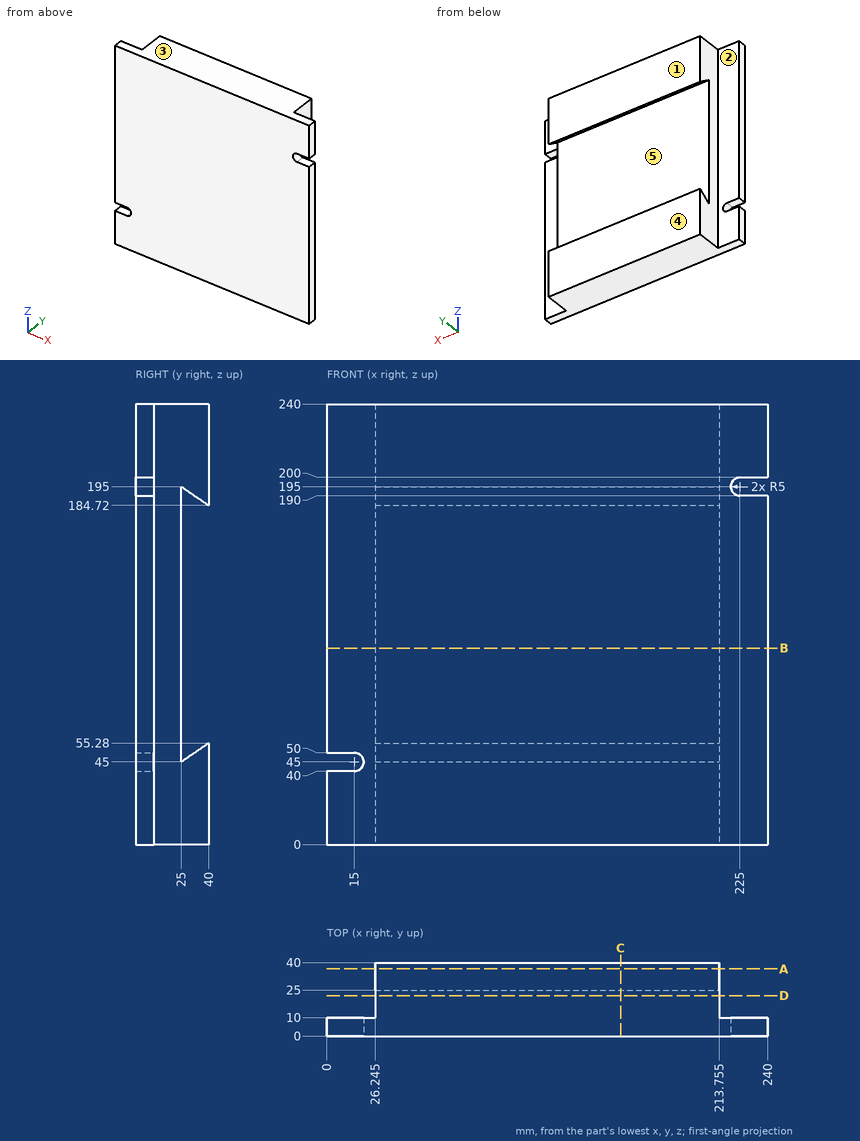
Part print with two shaded views. Sizes in mm from the minimum x, y, z corner. A direction names the side the tool comes from. Round coordinates to 2 decimals unless told otherwise and drop trailing zeros. Write each loop counter-clockwise with the first axis right and the second up, starting at its lowest first coordinate (ties: lowest second). Pieces come first, ordered by that corner, then holes. Notation, with made-up numbers: (-29, 39) -> (4, 39) arc R25 cw to (4, 75) -> close; hole circle Ø5 at (19.25, 34.5). An arc over 180 degrees is marked (long way). Put each result on its own line as item: value.
Item 1: Flat gauge pins, fed straight in: P1, Ø9, axis at y = 21.5, z = 108.5, coming from the -X side (1 decimal); P2, Ø13, axis at x = 14, z = 167, coming from the +Y side; P3, Ø1.5, axis at y = 17.5, z = 121, coming from the +X side (1 decimal). Where does each tip first touch, or does it go through?
Here are the results:
P1: stops at x = 26.2
P2: stops at y = 10
P3: stops at x = 213.8
Item 2: Two-plate mould, pull along Z, no slides. Class the marked faces 3, 4 and 5: pulls with the +Z half, pulls with the -Z half, needs draft (parallel to the pull), parting line crosses it, or undercut.
Here are the results:
face 3: pulls with the +Z half
face 4: needs draft
face 5: undercut
Item 3: Slice it at C-C, the plane x = 160. Give the cut face in (y, z), plus the area to 3 significant figures.
Here are the results:
outline: (0, 0) -> (40, 0) -> (40, 55.28) -> (25, 45) -> (25, 195) -> (40, 184.72) -> (40, 240) -> (0, 240) -> close
area: 7,500 mm^2
Item 4: Slice it at A-A, the plane y = 36.5. Give the cut face in (x, z) (1 decimal), plus the area to 3 significant figures.
Here are the results:
outline: (26.2, 0) -> (213.8, 0) -> (213.8, 52.9) -> (26.2, 52.9) -> close; (26.2, 187.1) -> (213.8, 187.1) -> (213.8, 240) -> (26.2, 240) -> close
area: 19,800 mm^2
Item 5: Wall check: probe 1 along X at (y, z) = (23, 204) (1 decimal); probe 2 along Z at (x, y) = (81, 35); probe 3 along Y at (x, z) = (111, 56). Give the ranges that are in metal, low to high. Write a range as from..to.
Here are the results:
probe 1: x = 26.2..213.8
probe 2: z = 0..51.85, 188.15..240
probe 3: y = 0..25
Item 6: Slice it at D-D, the plane y = 22. Give the cut face in (x, z) (1 decimal).
Here are the results:
outline: (26.2, 0) -> (213.8, 0) -> (213.8, 240) -> (26.2, 240) -> close
Item 7: Tool access for the marked faces 1 and 2: list every direction of +Z, -Z, +X, -X, +Y, -Y with a clear straight run to the whole face (end or side of a thin tool).
Here are the results:
face 1: +Z, -Z, +X, -X, +Y
face 2: +Z, -Z, -X, +Y
Item 8: Slice it at B-B, the plane z = 107. Give the cut face in (x, y) (1 decimal).
Here are the results:
outline: (0, 0) -> (240, 0) -> (240, 10) -> (213.8, 10) -> (213.8, 25) -> (26.2, 25) -> (26.2, 10) -> (0, 10) -> close
